Input: part model. Units: mm. Frame: model coordinates. Face numbers are marked on the shaded views. A direction names the side the tool comes from. Give positions to 0.01 mm unless a question says otherwise; leave off trailing zeros. Order: outer loops, then holes, each group sorted by start corner. A loop starts at its lowest first (then second) coordinate and runs counter-clockwise, first axis right, second up. Notation, with made-up numbers: M 52,68 L 96,68 A16 cw 96,87 Z; hole C 87.5,20.5 d5. An arc over 180 degrees is marked long. Use a Markdown table: item, result.
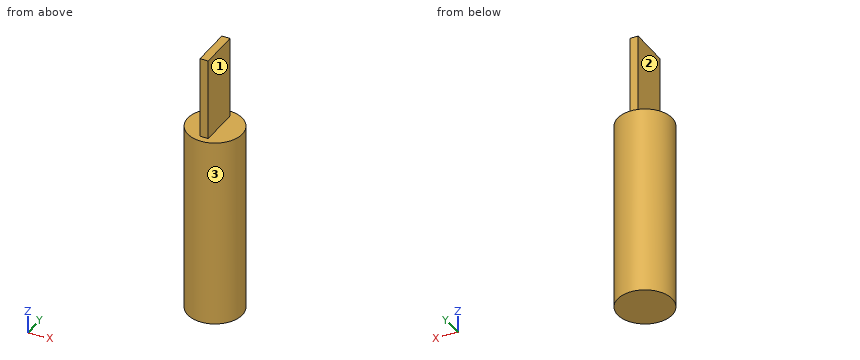
from build123d import *

# Parameters (mm, degrees)
F2_W     = 3
F2_H     = 15
F0_DEPTH = 100
F2_R     = 10
F1_DEPTH = 70


with BuildPart() as f0:
    # F2 (on Top) → F0 (new body)
    with BuildSketch(Plane.XY):
        Rectangle(F2_W, F2_H)
    extrude(amount=F0_DEPTH)

    # F2 (on Top) → F1 (join)
    with BuildSketch(Plane.XY):
        Circle(F2_R)
        Rectangle(F2_W, F2_H, mode=Mode.SUBTRACT)
    extrude(amount=F1_DEPTH)


solid = f0.part
1) Material intervals for line 1 (X direction, y = -6.75, z = 90); line 2 (Z direction, x = 7.5, y = -1); line 3 (Y direction, x = 0.75, z = 94), sorted ascending. Write a range as from..to.
Response values:
| item | result |
|---|---|
| line 1 | x = -1.5..1.5 |
| line 2 | z = 0..70 |
| line 3 | y = -7.5..7.5 |
2) First-contact query: pin 1 Ø5 at (x, z) = (-2.5, 79.5) entering from +Y; pin 2 Ø5 at (y, z) = (-3.5, 60.5) entering from -X; pin 3 Ø7.5 at (y, z) = (-2.5, 88) entering from -X. Flat tips, straight axial feed; report the tip coordinate or a pass-through.
Response values:
| item | result |
|---|---|
| pin 1 | stops at y = 7.5 |
| pin 2 | stops at x = -9.95 |
| pin 3 | stops at x = -1.5 |
3) Cut plane A-A on y = 0. Return loops of the section in (x, z), and give its area (3 significant figures).
Response values:
| item | result |
|---|---|
| outline | M -10,0 L 10,0 L 10,70 L 1.5,70 L 1.5,100 L -1.5,100 L -1.5,70 L -10,70 Z |
| area | 1,490 mm² |
4) Cut plane D-D on x = 6.5. Return loops of the section in (y, z), and give its area (3 significant figures).
Response values:
| item | result |
|---|---|
| outline | M -7.6,0 L 7.6,0 L 7.6,70 L -7.6,70 Z |
| area | 1,060 mm² |
5) Reachability of the marked faces 1, 2 and 3 from +Z, -Z, +X, -X, +Y, -Y: full face, straight path, thin tool, end or side. Return the list, or none.
Response values:
| item | result |
|---|---|
| face 1 | +Z, +X, +Y, -Y |
| face 2 | +Z, -X, +Y, -Y |
| face 3 | +Z, -Z |
6) Cut plane B-B on x = 0. Return loops of the section in (y, z).
Response values:
| item | result |
|---|---|
| outline | M -10,0 L 10,0 L 10,70 L 7.5,70 L 7.5,100 L -7.5,100 L -7.5,70 L -10,70 Z |
7) Cut plane C-C on z = 88.5. Return loops of the section in (x, y), and give its area (3 significant figures).
Response values:
| item | result |
|---|---|
| outline | M -1.5,-7.5 L 1.5,-7.5 L 1.5,7.5 L -1.5,7.5 Z |
| area | 45.0 mm² |
